Part print with two shaded views. Sizes in mm from the minimum x, y, z corner. A direction names the side the tool comes from. Coordinates: 2 decimals unless noted, no trailing zeros. Write each loop counter-clockwise with the first axis right and the second up, starting at its lowest first coordinate (ties: lowest second). Pieces come first, ordered by that corner, then holes.
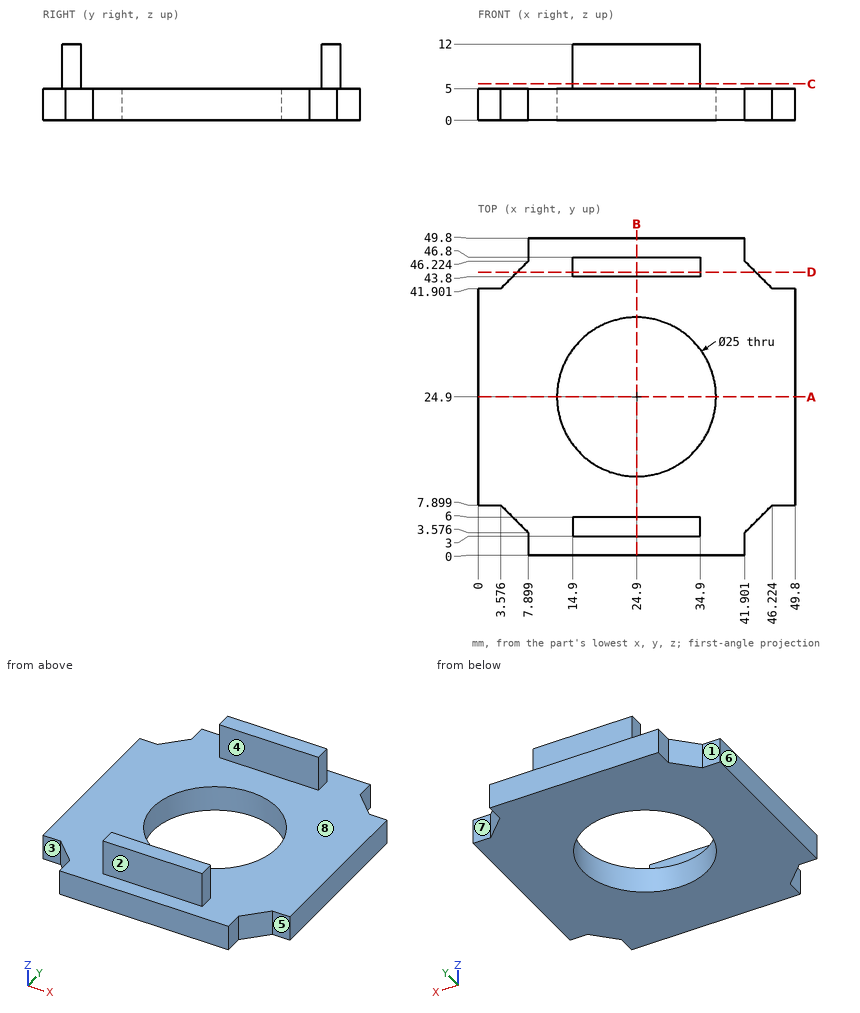
(1) Slice it at D-D, the plane y = 44.5. List the corners of the cut face in (x, z) (1 decimal), and give its area (3 significant figures).
(2) Slice it at A-A, the plane y = 24.9. List the corners of the cut face in (x, z), and give its area (3 significant figures).
(3) Two-plate mould, pull along Y, no slides. Class the marked faces 6, 7 and 8: pulls with the +Y half, pulls with the -Y half, needs draft (parallel to the pull), parting line crosses it, or undercut.
(4) 3-axis set-ups, long thin cutter, end or side, ignore diameter. For the marked faces 1, 2, 3, 4 and 5: which of +Z, -Z, +X, -X, +Y, -Y reach the whole face in a straight line?
(5) Slice it at B-B, the plane x = 24.9. List the corners of the cut face in (y, z).
(6) Probe L1, parallel to Y at x = 24.9, z = 1.8; L2, parallel to Y at x = 17.5, z = 8; L3, parallel to Z at x = 21, y = 10. List the from-to ranges inside material, lowest first.
(7) Slice it at C-C, the plane z = 5.75. List the corners of the cut face in (x, y), and give its area (3 significant figures).
(8) Flat gauge pins, fed straight in: P1, Ø4, axis at x = 1.5, z = 3.5, coming from the +Y side; P2, Ø6, axis at y = 6, z = 6, coming from the -X side; P3, Ø1.5, axis at x = 44.5, z = 1.5, coming from the +Y side (1 decimal); P4, Ø1.5, axis at y = 4.5, z = 8.5, coming from the +X side. Where does each tip first touch, or does it go through?
Results:
1. outline: (6.2, 0) - (43.6, 0) - (43.6, 5) - (34.9, 5) - (34.9, 12) - (14.9, 12) - (14.9, 5) - (6.2, 5) - close
1. area: 327 mm2
2. outline: (0, 0) - (12.4, 0) - (12.4, 5) - (0, 5) - close; (37.4, 0) - (49.8, 0) - (49.8, 5) - (37.4, 5) - close
2. area: 124 mm2
3. face 6: needs draft
3. face 7: pulls with the +Y half
3. face 8: undercut
4. face 1: +Z, -Z, -X, +Y
4. face 2: +Z, +X, -X, -Y
4. face 3: +Z, -Z, -X, -Y
4. face 4: +Z, +X, -X
4. face 5: +Z, -Z, +X, -Y
5. outline: (0, 0) - (12.4, 0) - (12.4, 5) - (6, 5) - (6, 12) - (3, 12) - (3, 5) - (0, 5) - close; (37.4, 0) - (49.8, 0) - (49.8, 5) - (46.8, 5) - (46.8, 12) - (43.8, 12) - (43.8, 5) - (37.4, 5) - close
6. L1: y = 0 to 12.4, 37.4 to 49.8
6. L2: y = 3 to 6, 43.8 to 46.8
6. L3: z = 0 to 5
7. outline: (14.9, 3) - (34.9, 3) - (34.9, 6) - (14.9, 6) - close; (14.9, 43.8) - (34.9, 43.8) - (34.9, 46.8) - (14.9, 46.8) - close
7. area: 120 mm2
8. P1: stops at y = 41.9
8. P2: stops at x = 0
8. P3: stops at y = 44.4
8. P4: stops at x = 34.9
